```python
from build123d import *

# Parameters (mm, degrees)
SKETCH_1_R               = 8
EXTRUDE_1_DEPTH          = 2
EXTRUDE_START            = 2
SKETCH_1_3_R             = 1.25
EXTRUDE_2_DEPTH          = 3
SKETCH_2_R               = 5
SKETCH_2_R_2             = 1.5
EXTRUDE_3_DEPTH          = 0.01
SKETCH_3_R               = 3.25
SKETCH_3_R_2             = 2.45
EXTRUDE_4_DEPTH          = 8
CUT_EXTRUDE_1_DEPTH      = 14.862182368
CUT_EXTRUDE_1_DEPTH_BACK = 14.862182368
SKETCH_2_2_R             = 1.5
CUT_EXTRUDE_2_REACH      = 17.106


with BuildPart() as part:
    # 草图1 → 凸台-拉伸1 (new body)
    with BuildSketch(Plane(origin=(0, 0, 0), x_dir=(0, 0, -1), z_dir=(1, 0, 0))):
        Circle(SKETCH_1_R)
    extrude(amount=EXTRUDE_1_DEPTH)

    # 草图1<3> → 凸台-拉伸2 (add)
    with BuildSketch(Plane(origin=(0, 0, 0), x_dir=(0, 0, -1), z_dir=(1, 0, 0)).offset(EXTRUDE_START)):
        with Locations((0, 6.25)):
            Circle(SKETCH_1_3_R)
        with Locations((-5.412658774, -3.125)):
            Circle(SKETCH_1_3_R)
        with Locations((5.412658774, -3.125)):
            Circle(SKETCH_1_3_R)
    extrude(amount=EXTRUDE_2_DEPTH)

    # 草图2 → 凸台-拉伸3 (add)
    with BuildSketch(Plane.ZY):
        with Locations(Location((0, 0, 0), (0, 0, 180))):
            Circle(SKETCH_2_R)
        with Locations(Location((0, 0, 0), (0, 0, 180))):
            Circle(SKETCH_2_R_2, mode=Mode.SUBTRACT)
    extrude(amount=EXTRUDE_3_DEPTH)

    # 草图3 → 凸台-拉伸4 (add)
    # profile 1 of 5: a face of its own
    with BuildSketch(Plane.ZY.offset(0.01)):
        Circle(SKETCH_3_R)
        Circle(SKETCH_3_R_2, mode=Mode.SUBTRACT)
    # profile 2 of 5: a face of its own
    with BuildSketch(Plane.ZY.offset(0.01)):
        with BuildLine():
            ThreePointArc((-1.092787266, 2.192787266), (-1.732411614, 1.732411614), (-2.192787266, 1.092787266))
            Line((-2.192787266, 1.092787266), (-1.092787266, 1.092787266))
            Line((-1.092787266, 1.092787266), (-1.092787266, 2.192787266))
        make_face()
    # profile 3 of 5: a face of its own
    with BuildSketch(Plane.ZY.offset(0.01)):
        with BuildLine():
            Line((-1.092787266, -1.092787266), (-2.192787266, -1.092787266))
            ThreePointArc((-2.192787266, -1.092787266), (-1.732411614, -1.732411614), (-1.092787266, -2.192787266))
            Line((-1.092787266, -2.192787266), (-1.092787266, -1.092787266))
        make_face()
    # profile 4 of 5: a face of its own
    with BuildSketch(Plane.ZY.offset(0.01)):
        with BuildLine():
            Line((2.192787266, -1.092787266), (1.092787266, -1.092787266))
            Line((1.092787266, -1.092787266), (1.092787266, -2.192787266))
            ThreePointArc((1.092787266, -2.192787266), (1.732411614, -1.732411614), (2.192787266, -1.092787266))
        make_face()
    # profile 5 of 5: a face of its own
    with BuildSketch(Plane.ZY.offset(0.01)):
        with BuildLine():
            Line((1.092787266, 2.192787266), (1.092787266, 1.092787266))
            Line((1.092787266, 1.092787266), (2.192787266, 1.092787266))
            ThreePointArc((2.192787266, 1.092787266), (1.732411614, 1.732411614), (1.092787266, 2.192787266))
        make_face()
    extrude(amount=EXTRUDE_4_DEPTH)

    # 草图2<2> → 切除-拉伸1 (cut, two sides: drawn at the far end of the back side and taken through both)
    with BuildSketch(Plane.ZY.offset(-CUT_EXTRUDE_1_DEPTH_BACK)):
        with Locations(Location((0, 0, 0), (0, 0, 180))):
            Circle(SKETCH_2_2_R)
    extrude(amount=CUT_EXTRUDE_1_DEPTH + CUT_EXTRUDE_1_DEPTH_BACK, mode=Mode.SUBTRACT)

    # 切除-拉伸2: up to this face of the body (flat: up to its plane)
    cut_extrude_2_end = Plane(part.part.faces().sort_by_distance((-0.01, 0, 4.858578644))[0])
    # 草图4 → 切除-拉伸2 (cut, up to the picked face)
    with BuildSketch(Plane(origin=(2, 0, 0), x_dir=(0, 0, -1), z_dir=(1, 0, 0)), mode=Mode.PRIVATE) as cut_extrude_2_sk1:
        with BuildLine():
            Line((-2, 1.154700538), (-2, 4.85412196))
            ThreePointArc((-2, 4.85412196), (-4.54663337, 2.625), (-5.20379293, -0.695010172))
            Line((-5.20379293, -0.695010172), (-2, 1.154700538))
        make_face()
    cut_extrude_2_tool1 = split(extrude(cut_extrude_2_sk1.sketch, amount=-CUT_EXTRUDE_2_REACH, mode=Mode.PRIVATE), bisect_by=cut_extrude_2_end, keep=Keep.BOTH, mode=Mode.PRIVATE)
    # 草图4 → 切除-拉伸2 (cut, up to the picked face)
    with BuildSketch(Plane(origin=(2, 0, 0), x_dir=(0, 0, -1), z_dir=(1, 0, 0)), mode=Mode.PRIVATE) as cut_extrude_2_sk2:
        with BuildLine():
            Line((2, 1.154700538), (5.20379293, -0.695010172))
            ThreePointArc((5.20379293, -0.695010172), (5.238435496, -0.348272247), (5.25, 0))
            ThreePointArc((5.25, 0), (4.362482092, 2.920830361), (2, 4.85412196))
            Line((2, 4.85412196), (2, 1.154700538))
        make_face()
    cut_extrude_2_tool2 = split(extrude(cut_extrude_2_sk2.sketch, amount=-CUT_EXTRUDE_2_REACH, mode=Mode.PRIVATE), bisect_by=cut_extrude_2_end, keep=Keep.BOTH, mode=Mode.PRIVATE)
    # 草图4 → 切除-拉伸2 (cut, up to the picked face)
    with BuildSketch(Plane(origin=(2, 0, 0), x_dir=(0, 0, -1), z_dir=(1, 0, 0)), mode=Mode.PRIVATE) as cut_extrude_2_sk3:
        with BuildLine():
            ThreePointArc((-3.20379293, -4.159111787), (0, -5.25), (3.20379293, -4.159111787))
            Line((3.20379293, -4.159111787), (0, -2.309401077))
            Line((0, -2.309401077), (-3.20379293, -4.159111787))
        make_face()
    cut_extrude_2_tool3 = split(extrude(cut_extrude_2_sk3.sketch, amount=-CUT_EXTRUDE_2_REACH, mode=Mode.PRIVATE), bisect_by=cut_extrude_2_end, keep=Keep.BOTH, mode=Mode.PRIVATE)
    # 草图4 → 切除-拉伸2 (cut, up to the picked face)
    with BuildSketch(Plane(origin=(2, 0, 0), x_dir=(0, 0, -1), z_dir=(1, 0, 0)), mode=Mode.PRIVATE) as cut_extrude_2_sk4:
        with BuildLine():
            ThreePointArc((-2, 7.745966692), (-6.92820323, 4), (-7.708203932, -2.140932539))
            Line((-7.708203932, -2.140932539), (-7.035053852, -1.752289159))
            ThreePointArc((-7.035053852, -1.752289159), (-6.278684177, 3.625), (-2, 6.968679932))
            Line((-2, 6.968679932), (-2, 7.745966692))
        make_face()
    cut_extrude_2_tool4 = split(extrude(cut_extrude_2_sk4.sketch, amount=-CUT_EXTRUDE_2_REACH, mode=Mode.PRIVATE), bisect_by=cut_extrude_2_end, keep=Keep.BOTH, mode=Mode.PRIVATE)
    # 草图4 → 切除-拉伸2 (cut, up to the picked face)
    with BuildSketch(Plane(origin=(2, 0, 0), x_dir=(0, 0, -1), z_dir=(1, 0, 0)), mode=Mode.PRIVATE) as cut_extrude_2_sk5:
        with BuildLine():
            Line((7.035053852, -1.752289159), (7.708203932, -2.140932539))
            ThreePointArc((7.708203932, -2.140932539), (7.926715318, -1.080363027), (8, 0))
            ThreePointArc((8, 0), (6.32455532, 4.898979486), (2, 7.745966692))
            Line((2, 7.745966692), (2, 6.968679932))
            ThreePointArc((2, 6.968679932), (5.790617411, 4.362482092), (7.25, 0))
            ThreePointArc((7.25, 0), (7.196062827, -0.882711609), (7.035053852, -1.752289159))
        make_face()
    cut_extrude_2_tool5 = split(extrude(cut_extrude_2_sk5.sketch, amount=-CUT_EXTRUDE_2_REACH, mode=Mode.PRIVATE), bisect_by=cut_extrude_2_end, keep=Keep.BOTH, mode=Mode.PRIVATE)
    # 草图4 → 切除-拉伸2 (cut, up to the picked face)
    with BuildSketch(Plane(origin=(2, 0, 0), x_dir=(0, 0, -1), z_dir=(1, 0, 0)), mode=Mode.PRIVATE) as cut_extrude_2_sk6:
        with BuildLine():
            ThreePointArc((-5.708203932, -5.605034154), (0, -8), (5.708203932, -5.605034154))
            Line((5.708203932, -5.605034154), (5.035053852, -5.216390774))
            ThreePointArc((5.035053852, -5.216390774), (0, -7.25), (-5.035053852, -5.216390774))
            Line((-5.035053852, -5.216390774), (-5.708203932, -5.605034154))
        make_face()
    cut_extrude_2_tool6 = split(extrude(cut_extrude_2_sk6.sketch, amount=-CUT_EXTRUDE_2_REACH, mode=Mode.PRIVATE), bisect_by=cut_extrude_2_end, keep=Keep.BOTH, mode=Mode.PRIVATE)
    add(cut_extrude_2_tool1.solids().sort_by(Axis((2, 2.006872, 3.476004), (-1, 0, 0)))[0], mode=Mode.SUBTRACT)
    add(cut_extrude_2_tool2.solids().sort_by(Axis((2, 2.006872, -3.476004), (-1, 0, 0)))[0], mode=Mode.SUBTRACT)
    add(cut_extrude_2_tool3.solids().sort_by(Axis((2, -4.013743, 0), (-1, 0, 0)))[0], mode=Mode.SUBTRACT)
    add(cut_extrude_2_tool4.solids().sort_by(Axis((2, 7.357323, 2.115651), (-1, 0, 0)))[0], mode=Mode.SUBTRACT)
    add(cut_extrude_2_tool5.solids().sort_by(Axis((2, -1.846454, -7.429454), (-1, 0, 0)))[0], mode=Mode.SUBTRACT)
    add(cut_extrude_2_tool6.solids().sort_by(Axis((2, -7.367509, 0), (-1, 0, 0)))[0], mode=Mode.SUBTRACT)


solid = part.part
```
The model under review builds one solid part; all positions refer to its coordinate system, in mm. A direction names the side the tool comes from. Give positions to 0.01 mm unless a question says otherwise; leave off trailing zeros. Loops run counter-clockwise (first coordinate to the right, second up) from the corner with the lowest first, then second, coordinate; pieces in that order, holes last. Notation, with made-up numbers: (30, 56.5) - (46, 56.5) arc R23 cw to (46, 93.5) - close; hole circle Ø6 at (19, 59). An arc over 180 degrees is marked (long way). Answer as a JSON object with one key per item and string values.
Q1. Insertion check: pin 1 (1.6 mm diameter, centred on x = 0.5, y = 2.5, fed in from -Z); pin 2 (0.9 mm diameter, centred on x = -3, z = -1.5, fed in from +Y); pin 3 (1.5 mm diameter, centred on y = -0.5, z = 0, fed in from -X) (3 decimals); pin 4 (0.5 mm diameter, centred on x = -4.5, y = -1.5, fed in from +Z). Each pin has a flat end and moves straight along its axis. Give the tip position at first contact, or say it passes through.
Worked out:
{"pin 1": "stops at z = -7.05", "pin 2": "stops at y = 3.08", "pin 3": "passes through", "pin 4": "stops at z = 3"}
Q2. Add section B-B on x = 1.25. State the section outline as (y, z) points.
Worked out:
{"outline": "(-5.61, -5.71) arc R8 ccw to (-2.14, -7.71) - (-1.75, -7.04) arc R7.25 ccw to (6.97, -2) - (7.75, -2) arc R8 ccw to (7.75, 2) - (6.97, 2) arc R7.25 ccw to (-1.75, 7.04) - (-2.14, 7.71) arc R8 ccw to (-5.61, 5.71) - (-5.22, 5.04) arc R7.25 ccw to (-5.22, -5.04) - close; hole (-4.16, -3.2) - (-2.31, 0) - (-4.16, 3.2) arc R5.25 ccw to start; hole circle Ø3 at (0, 0); hole (-0.7, -5.2) arc R5.25 ccw to (4.85, -2) - (1.15, -2) - close; hole (-0.7, 5.2) - (1.15, 2) - (4.85, 2) arc R5.25 ccw to start"}
Q3. For faces 1 (the cylindrical face through (-3.954, -1.978, -2.579)), 2 (the cylindrical face through (1.01, -7.25, -0.08)), list the 3-axis set-ups (+Z, -Z, +X, -X, +Y, -Y) from which the entire face can be reached by the end or side of a thin tool; tool diameter is ignored.
Worked out:
{"face 1": "-X", "face 2": "+X, -X, -Y"}
Q4. Add section A-A on x = -4.75. State the section outline as (y, z) points.
Worked out:
{"outline": "circle Ø6.5 at (0, 0); hole (-2.19, -1.09) - (-1.09, -1.09) - (-1.09, -2.19) arc R2.45 ccw to (1.09, -2.19) - (1.09, -1.09) - (2.19, -1.09) arc R2.45 ccw to (2.19, 1.09) - (1.09, 1.09) - (1.09, 2.19) arc R2.45 ccw to (-1.09, 2.19) - (-1.09, 1.09) - (-2.19, 1.09) arc R2.45 ccw to start"}
Q5. Mouldability with a two-part tool opening along Z and no side actions: class faces 3 (the flat face through (-4, 2, 1.093)), 4 (the cylindrical face through (1.014, 3.557, 6.317)), 5 (the flat face through (-0.01, -2, 4)), 6 (the cylindrical face through (1.01, 2.67, 4.52)) as +Z half, -Z half, draft (parallel to the pull), parting line (faces both ways), or undercut.
Worked out:
{"face 3": "undercut", "face 4": "+Z half", "face 5": "draft", "face 6": "undercut"}
Q6. To check wall thickness, follow line 1 along Z through (x, y) = (1.25, 3.25); line 2 along X through (y, z) = (2.5, 1.75); line 3 along Y through (x, z) = (0.25, -4). State the ranges of each line that lie inside material, in increasing order.
Worked out:
{"line 1": "z = -6.48 to -4.12, -2 to 2, 4.12 to 6.48", "line 2": "x = -8.01 to 2", "line 3": "y = -6.05 to 0, 3.4 to 6.05"}
Q7. Add section D-D on y = 3.75. State the section outline as (x, z) points, plus the area to 3 significant figures.
Worked out:
{"outline": "(-0.01, -2) - (2, -2) - (2, 2) - (-0.01, 2) - close; (0, -6.2) - (2, -6.2) - (2, -3.67) - (0, -3.67) - close; (0, 3.67) - (2, 3.67) - (2, 6.2) - (0, 6.2) - close", "area": "18.2 mm^2"}
